Geometry check sheet. Reference: the model listing, model coordinates, mm. A direction names the side the tool comes from. Coordinates: 2 decimals unless noted, no trailing zeros. Loops run counter-clockwise (first coordinate to the right, second up) from the corner with the lowest first, then second, coordinate; pieces in that order, holes last. Notation, with made-up numbers: (-13, 17) - (11, 17) arc R18 ccw to (11, 52) - close; hole circle Ø6 at (21.5, 79.5). An arc over 180 degrees is marked (long way). One line per item, written item: value.
from build123d import *

# Parameters (mm, degrees)
CROQUIS1_R              = 31.5
SALIENTE_EXTRUIR1_DEPTH = 2.4
CROQUIS2_W              = 16.1
CROQUIS2_H              = 36.6
CROQUIS2_W_2            = 12.5
CROQUIS2_H_2            = 33
SALIENTE_EXTRUIR2_DEPTH = 22.5
CROQUIS5_W              = 16.1
CROQUIS5_H              = 36.6
CORTAR_EXTRUIR2_DEPTH   = 9
CROQUIS6_R              = 1.5
CORTAR_EXTRUIR3_DEPTH   = 2.4
CROQUIS7_W              = 12.5
CROQUIS7_H              = 9
SALIENTE_EXTRUIR3_DEPTH = 33
CROQUIS8_R              = 1
CORTAR_EXTRUIR5_DEPTH   = 9
SALIENTE_EXTRUIR4_DEPTH = 12.5
CROQUIS10_W             = 4
CROQUIS10_H             = 2
CORTAR_EXTRUIR6_DEPTH   = 9
SALIENTE_EXTRUIR5_DEPTH = 2.4
SALIENTE_EXTRUIR6_DEPTH = 16.1
CORTAR_EXTRUIR7_DEPTH   = 1.8
CROQUIS14_R             = 1.5
SALIENTE_EXTRUIR7_DEPTH = 0.6


with BuildPart() as part:
    # Croquis1 → Saliente-Extruir1 (new body)
    with BuildSketch(Plane.XY):
        with Locations((-51.235671923, 9.786589019)):
            Circle(CROQUIS1_R)
    extrude(amount=SALIENTE_EXTRUIR1_DEPTH)

    # Croquis2 → Saliente-Extruir2 (add)
    with BuildSketch(Plane.XY.offset(2.4)):
        with Locations((-51.235671923, 6.086589019)):
            Rectangle(CROQUIS2_W, CROQUIS2_H)
        with Locations((-51.235671923, 6.086589019)):
            Rectangle(CROQUIS2_W_2, CROQUIS2_H_2, mode=Mode.SUBTRACT)
    extrude(amount=SALIENTE_EXTRUIR2_DEPTH)

    # Croquis5 → Cortar-Extruir2 (cut)
    with BuildSketch(Plane.XY.offset(2.4)):
        with Locations((-51.235671923, 6.086589019)):
            Rectangle(CROQUIS5_W, CROQUIS5_H)
    extrude(amount=-CORTAR_EXTRUIR2_DEPTH, mode=Mode.SUBTRACT)


with BuildPart() as cortar_extruir2_piece_1:
    # of the separate pieces the step leaves, piece 1, a body of its own (cortar_extruir2_pieces)
    add(part.part.solids().sort_by_distance((-19.735671923, 9.786589019, 0))[0])

    # Croquis6 → Cortar-Extruir3 (cut)
    with BuildSketch(Plane(origin=(0, 0, 0), x_dir=(-1, 0, 0), z_dir=(0, 0, -1))):
        with Locations((34.618662565, 26.403598377)):
            Circle(CROQUIS6_R)
        with Locations((67.85268128, 26.403598377)):
            Circle(CROQUIS6_R)
        with Locations((67.85268128, -6.830420339)):
            Circle(CROQUIS6_R)
        with Locations((34.618662565, -6.830420339)):
            Circle(CROQUIS6_R)
        Polygon((51.235671923, 24.386589019), (53.235671923, 24.386589019), (53.235671923, 44.386589019), (49.235671923, 44.386589019), (49.235671923, 24.386589019), align=None)
    extrude(amount=-CORTAR_EXTRUIR3_DEPTH, mode=Mode.SUBTRACT)



with BuildPart() as cortar_extruir2_piece_2:
    # of the separate pieces the step leaves, piece 2, a body of its own (cortar_extruir2_pieces)
    add(part.part.solids().sort_by_distance((-59.285671923, -12.213410981, 24.9))[0])

    # Croquis7 → Saliente-Extruir3 (add)
    with BuildSketch(Plane.XZ.offset(-22.586589019)):
        with Locations((-51.235671923, 13.4)):
            Rectangle(CROQUIS7_W, CROQUIS7_H)
    extrude(amount=SALIENTE_EXTRUIR3_DEPTH)

    # Croquis8 → Cortar-Extruir5 (cut)
    with BuildSketch(Plane.XY.offset(17.9)):
        with Locations((-51.235671923, -8.413410981)):
            Circle(CROQUIS8_R)
        with Locations((-51.235671923, 20.636589019)):
            Circle(CROQUIS8_R)
        Polygon((-44.985671923, -5.413410981), (-57.485671923, -5.413410981), (-57.485671923, 17.586589019), (-53.235671923, 17.586589019), (-53.235671923, 19.586589019), (-49.235671923, 19.586589019), (-49.235671923, 17.586589019), (-44.985671923, 17.586589019), align=None)
    extrude(amount=-CORTAR_EXTRUIR5_DEPTH, mode=Mode.SUBTRACT)

    # Croquis9 → Saliente-Extruir4 (add)
    with BuildSketch(Plane.ZY.offset(44.985671923)):
        Polygon((8.9, -5.413410981), (3.9, -10.413410981), (8.9, -10.413410981), align=None)
        Polygon((8.9, 17.586589019), (3.9, 22.586589019), (8.9, 22.586589019), align=None)
    extrude(amount=SALIENTE_EXTRUIR4_DEPTH)

    # Croquis10 → Cortar-Extruir6 (cut)
    with BuildSketch(Plane.XY.offset(8.9)):
        with Locations((-51.235671923, 18.586589019)):
            Rectangle(CROQUIS10_W, CROQUIS10_H)
    extrude(amount=-CORTAR_EXTRUIR6_DEPTH, mode=Mode.SUBTRACT)


with BuildPart() as cortar_extruir2_piece_1_1:
    add(cortar_extruir2_piece_1.part)

    add(cortar_extruir2_piece_2.part)  # Saliente-Extruir5 merges Cortar-Extruir2 piece 2
    # Croquis11 → Saliente-Extruir5 (add)
    with BuildSketch(Plane(origin=(0, 0, 2.4), x_dir=(-1, 0, 0), z_dir=(0, 0, -1))):
        Polygon((49.235671923, 24.386589019), (43.185671923, 24.386589019), (43.185671923, -12.213410981), (59.285671923, -12.213410981), (59.285671923, 24.386589019), (53.235671923, 24.386589019), (53.235671923, 22.586589019), (57.485671923, 22.586589019), (57.485671923, 10.586589019), (44.985671923, 10.586589019), (44.985671923, 22.586589019), (49.235671923, 22.586589019), align=None)
    extrude(amount=SALIENTE_EXTRUIR5_DEPTH)

    # Croquis12 → Saliente-Extruir6 (add)
    with BuildSketch(Plane(origin=(-43.185671923, 0, 0), x_dir=(0, 0, -1), z_dir=(1, 0, 0))):
        Polygon((-2.4, 24.386589019), (-7.4, 24.386589019), (-2.4, 29.386589019), align=None)
    extrude(amount=-SALIENTE_EXTRUIR6_DEPTH)

    # Croquis13 → Cortar-Extruir7 (cut)
    with BuildSketch(Plane.XY.offset(2.4)):
        Polygon((-31.385501057, -6.830420339), (-33.002081811, -4.030420339), (-36.235243318, -4.030420339), (-37.851824072, -6.830420339), (-36.235243318, -9.630420339), (-33.002081811, -9.630420339), align=None)
        Polygon((-64.619519773, -6.830420339), (-66.236100527, -4.030420339), (-69.469262034, -4.030420339), (-71.085842788, -6.830420339), (-69.469262034, -9.630420339), (-66.236100527, -9.630420339), align=None)
        Polygon((-37.851824072, 26.403598377), (-36.235243318, 23.603598377), (-33.002081811, 23.603598377), (-31.385501057, 26.403598377), (-33.002081811, 29.203598377), (-36.235243318, 29.203598377), align=None)
        Polygon((-71.085842788, 26.403598377), (-69.469262034, 23.603598377), (-66.236100527, 23.603598377), (-64.619519773, 26.403598377), (-66.236100527, 29.203598377), (-69.469262034, 29.203598377), align=None)
    extrude(amount=-CORTAR_EXTRUIR7_DEPTH, mode=Mode.SUBTRACT)

    # Croquis14 → Saliente-Extruir7 (add)
    with BuildSketch(Plane(origin=(0, 0, 0), x_dir=(-1, 0, 0), z_dir=(0, 0, -1))):
        with BuildLine():
            Line((53.235671923, 41.223032838), (53.235671923, 22.586589019))
            Line((53.235671923, 22.586589019), (57.485671923, 22.586589019))
            Line((57.485671923, 22.586589019), (57.485671923, 10.586589019))
            Line((57.485671923, 10.586589019), (44.985671923, 10.586589019))
            Line((44.985671923, 10.586589019), (44.985671923, 22.586589019))
            Line((44.985671923, 22.586589019), (49.235671923, 22.586589019))
            Line((49.235671923, 22.586589019), (49.235671923, 41.223032838))
            ThreePointArc((49.235671923, 41.223032838), (51.235671923, -21.713410981), (53.235671923, 41.223032838))
        make_face()
        with Locations((67.85268128, -6.830420339)):
            Circle(CROQUIS14_R, mode=Mode.SUBTRACT)
        with Locations((34.618662565, -6.830420339)):
            Circle(CROQUIS14_R, mode=Mode.SUBTRACT)
        with Locations((34.618662565, 26.403598377)):
            Circle(CROQUIS14_R, mode=Mode.SUBTRACT)
        with Locations((67.85268128, 26.403598377)):
            Circle(CROQUIS14_R, mode=Mode.SUBTRACT)
    extrude(amount=SALIENTE_EXTRUIR7_DEPTH)


solid = cortar_extruir2_piece_1_1.part
(1) Release check for a two-part mould opening along Y. For faces 1 (the face through (-51, -10.413, 3)), 2 (the face through (-49.879, -21.684, 0.921)), 3 (the face through (-51, 24.387, 16)) record: pulls with the +Y half, pulls with the -Y half, needs draft (parallel to the pull), parting line crosses it, or undercut.
Reply:
face 1: undercut
face 2: parting line crosses it
face 3: pulls with the +Y half
(2) Cross-section at C-C on x = -44. Record the cut outline in (y, z).
Reply:
outline: (-20.87, -0.6) - (40.44, -0.6) - (40.44, 2.4) - (29.39, 2.4) - (24.39, 7.4) - (24.39, 24.9) - (-12.21, 24.9) - (-12.21, 2.4) - (-20.87, 2.4) - close
(3) Material ranges on probe 1 along Y at (x, z) = (-49, 17); probe 2 along X at (y, z) = (-2.5, 7.75); probe 3 along Z at (x, y) = (-38, -10), recorded low to high. Write a range as from..to.
Reply:
probe 1: -12.21..-5.41, 17.59..24.39
probe 2: -59.29..-57.49, -44.99..-43.19
probe 3: -0.6..2.4
(4) Access from +Z, -Z, +X, -X, +Y, -Y to the whole of each face (thin tool, end or side, straight path). Record for faces 4 (the face through (-37.055, 25.023, 1.513)), 5 (the face through (-52, 19.587, 12)), 6 (the face through (-51, 22.587, 3)).
Reply:
face 4: +Z
face 5: +Z, -Z
face 6: -Z
(5) Cross-section at B-B on y = 18.5. Record the cut outline in (x, z), and give its area (3 significant figures).
Reply:
outline: (-81.51, -0.6) - (-57.49, -0.6) - (-57.49, 7.99) - (-53.24, 7.99) - (-53.24, 17.9) - (-57.49, 17.9) - (-57.49, 24.9) - (-59.29, 24.9) - (-59.29, 2.4) - (-81.51, 2.4) - close; (-49.24, 7.99) - (-44.99, 7.99) - (-44.99, -0.6) - (-20.96, -0.6) - (-20.96, 2.4) - (-43.19, 2.4) - (-43.19, 24.9) - (-44.99, 24.9) - (-44.99, 17.9) - (-49.24, 17.9) - close
area: 309 mm2
(6) Go/stop test with flat-tipped pins: pin 1 Ø3.5 at (x, z) = (-47.5, 15) entering from -Y; pin 2 Ø0.5 at (x, z) = (-68, 2) entering from -Y; pin 3 Ø4 at (y, z) = (-12.5, 21) entering from -X. Record where each tip stops, or that it passes through.
Reply:
pin 1: y = -12.21
pin 2: y = -17.04
pin 3: x = -59.29
(7) Cross-section at D-D on y = 7.5. Record the cut outline in (x, z).
Reply:
outline: (-82.65, -0.6) - (-19.82, -0.6) - (-19.82, 2.4) - (-43.19, 2.4) - (-43.19, 24.9) - (-44.99, 24.9) - (-44.99, 2.4) - (-57.49, 2.4) - (-57.49, 24.9) - (-59.29, 24.9) - (-59.29, 2.4) - (-82.65, 2.4) - close
(8) Cross-section at A-A on z = 23. Record the cut outline in (x, y), and give its area (3 significant figures).
Reply:
outline: (-59.29, -12.21) - (-43.19, -12.21) - (-43.19, 24.39) - (-59.29, 24.39) - close; hole (-57.49, -10.41) - (-44.99, -10.41) - (-44.99, 22.59) - (-57.49, 22.59) - close
area: 177 mm2
